Answer from the drawing. Dimensions are ordinates in mm from the lowest x, y and z of the part. Give positions to 0.01 mm unless a question says otherwise; leave off trailing zeros. Loops run counter-clockwise (first coordinate to the right, second up) from the corner with the lowest first, then second, coordinate; pieces in that order, holes last.
(1) This flat-tipped pin is pushed along its axis until it touches: P1, Ø1, axis at x = 3, y = 3.5, coming from the -Z side (1 decimal). Where does it stop, or does it pass through?
(2) Find section C-C, the plane y = 4.75. Write down the section's boundary in (x, z).
(3) Find section A-A, the plane z = 3.5. State how many separate pieces and enclosed holes the cut face has, then the cut area to 3 significant figures.
(4) Find section B-B, the plane x = 18.75. Write down the section's boundary in (y, z), then the cut area to 3 significant figures.
(5) Straight lines are drawn through the part: probe 1 along X at (y, z) = (1, 11); probe 2 along Y at (x, z) = (17, 3.7) (3 decimals); probe 3 along Z at (x, y) = (9.5, 3.5). For each, find the intervals that lie inside material, in ascending order.
(6) Find section D-D, the plane x = 12.75. Write down the section's boundary in (y, z), then the cut area to 3 significant figures.
(7) Determine the mould class of the marked faces 1, 2 and 3 for opening direction Z: pulls with the +Z half, pulls with the -Z half, needs draft (parallel to the pull), parting line crosses it, or undercut.
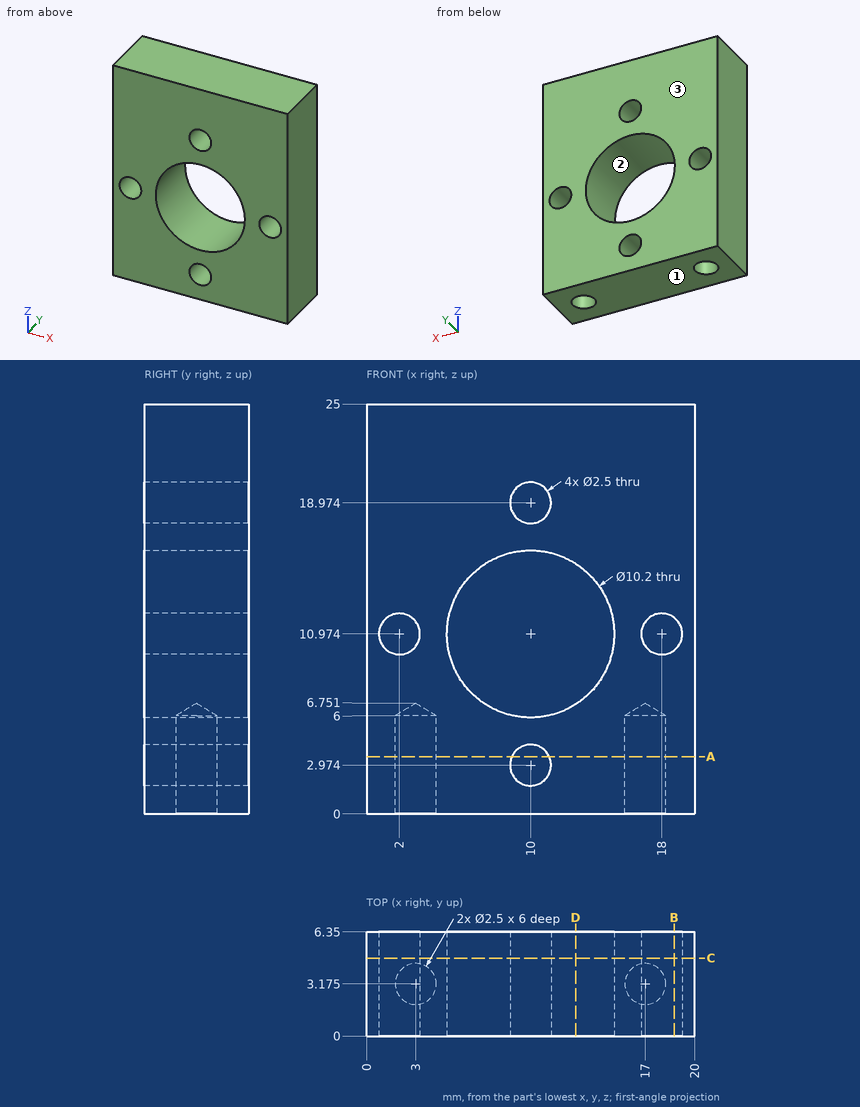
Entries:
1. P1: stops at z = 6.3
2. outline: (0, 0) - (20, 0) - (20, 25) - (0, 25) - close; hole circle Ø2.5 at (2, 10.97); hole circle Ø10.2 at (10, 10.97); hole circle Ø2.5 at (10, 2.97); hole circle Ø2.5 at (10, 18.97); hole circle Ø2.5 at (18, 10.97)
3. separate pieces: 2
3. enclosed holes: 2
3. area: 103 mm2
4. outline: (0, 0) - (6.35, 0) - (6.35, 9.97) - (0, 9.97) - close; (0, 11.97) - (6.35, 11.97) - (6.35, 25) - (0, 25) - close
4. area: 146 mm2
5. probe 1: x = 0 to 0.75, 3.25 to 4.9, 15.1 to 16.75, 19.25 to 20
5. probe 2: y = 0 to 1.925, 4.425 to 6.35
5. probe 3: z = 0 to 1.83, 4.12 to 5.9, 16.05 to 17.83, 20.12 to 25
6. outline: (0, 0) - (6.35, 0) - (6.35, 6.68) - (0, 6.68) - close; (0, 15.27) - (6.35, 15.27) - (6.35, 25) - (0, 25) - close
6. area: 104 mm2
7. face 1: pulls with the -Z half
7. face 2: undercut
7. face 3: needs draft
